Can you work these out from the model? Positions are in its coordinate system, mm. Face numbers are marked on the shaded views. A direction names the side the tool comes from. Give positions to 0.01 mm unless a question says otherwise; leave off trailing zeros. Loops run counter-clockwise (first coordinate to the right, second up) from the corner with the lowest first, then second, coordinate; pieces in that order, holes last. Notation, with made-up numbers: (85, 78.5) - (140, 78.5) arc R26 ccw to (140, 96.5) - close; hole circle Ø9 at (-25, 13). An arc over 180 degrees is marked (long way). Answer as a JSON object with one key per item and string values. Group by question number.
Item 1: Please list where these lines run through material, in increasing order: L1, parallel to Y at x = 9, z = 1.5; L2, parallel to Z at x = -45.5, y = -2.5; L3, parallel to Y at x = 9, z = 12.
Item 2: Suppose I cut it at C-C on x = -45.5. Write out the boundary of the cut face in (y, z), and give its area (3 significant figures).
Item 3: Which directions (+Z, -Z, +X, -X, +Y, -Y) give clear straight access to the entire face, cutting with the end or side of a thin tool? Please do the marked faces 1 and 2.
Item 4: Suppose I cut it at D-D on y = 13. Write out the boundary of the cut face in (x, z), and give its area (3 significant figures).
Item 5: Suppose I cut it at B-B on x = 20.5. Write out the boundary of the cut face in (y, z).
Item 6: Suppose I cut it at A-A on z = 26. Write out the boundary of the cut face in (x, y).
Item 7: Thinking about a two-plate mould opening in Y: for the marked faces 3, 4 and 5, which applies, pulls with the +Y half, pulls with the -Y half, needs draft (parallel to the pull), parting line crosses it, or undercut?
Item 8: Will these pins go through, and if not, where does the flat tip stop? pin 1 (6 mm diameter, centred on x = 16.5, z = 27, fed in from -Y); pin 2 (8 mm diameter, centred on x = -36, z = 26.5, fed in from +Y); pin 3 (1.5 mm diameter, centred on x = -15, y = -35, fed in from +Z).
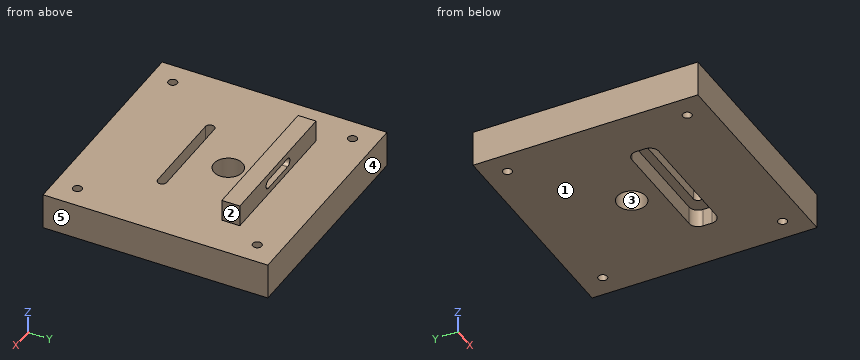
from build123d import *

# Parameters (mm, degrees)
SKETCH1_W           = 125
SKETCH1_H           = 125
BOSS_EXTRUDE1_DEPTH = 20
SKETCH2_R           = 2.5
CUT_EXTRUDE1_DEPTH  = 95.375743383
SKETCH3_R           = 8
CUT_EXTRUDE2_DEPTH  = 95.375743383
SKETCH4_W           = 70
SKETCH4_H           = 15
CUT_EXTRUDE3_DEPTH  = 10
FILLET1_R           = 5
SKETCH6_W           = 80
SKETCH6_H           = 10
BOSS_EXTRUDE2_DEPTH = 12
CUT_EXTRUDE4_DEPTH  = 123.375593875


with BuildPart() as part:
    # Sketch1 → Boss-Extrude1 (new body)
    with BuildSketch(Plane.XY):
        with Locations((4.174852652, 1.227897839)):
            Rectangle(SKETCH1_W, SKETCH1_H)
    extrude(amount=BOSS_EXTRUDE1_DEPTH)

    # Sketch2 → Cut-Extrude1 (cut, through all)
    with BuildSketch(Plane.XY.offset(20)):
        with Locations((-45.825147348, 51.227897839)):
            Circle(SKETCH2_R)
        with Locations((54.174852652, 51.227897839)):
            Circle(SKETCH2_R)
        with Locations((54.174852652, -48.772102161)):
            Circle(SKETCH2_R)
        with Locations((-45.825147348, -48.772102161)):
            Circle(SKETCH2_R)
    extrude(amount=-CUT_EXTRUDE1_DEPTH, mode=Mode.SUBTRACT)

    # Sketch3 → Cut-Extrude2 (cut, through all)
    with BuildSketch(Plane.XY.offset(20)):
        with Locations((4.174852652, 8.627897839)):
            Circle(SKETCH3_R)
        with BuildLine():
            Line((-20.825147348, -12.372102161), (29.174852652, -12.372102161))
            ThreePointArc((29.174852652, -12.372102161), (31.674852652, -14.872102161), (29.174852652, -17.372102161))
            Line((29.174852652, -17.372102161), (-20.825147348, -17.372102161))
            ThreePointArc((-20.825147348, -17.372102161), (-23.325147348, -14.872102161), (-20.825147348, -12.372102161))
        make_face()
    extrude(amount=-CUT_EXTRUDE2_DEPTH, mode=Mode.SUBTRACT)

    # Sketch4 → Cut-Extrude3 (cut)
    with BuildSketch(Plane(origin=(0, 0, 0), x_dir=(-1, 0, 0), z_dir=(0, 0, -1))):
        with Locations((-4.174852652, -14.872102161)):
            Rectangle(SKETCH4_W, SKETCH4_H)
    extrude(amount=-CUT_EXTRUDE3_DEPTH, mode=Mode.SUBTRACT)

    # Fillet1
    fillet1_edges = [part.edges().sort_by_distance(p)[0] for p in [
        (39.174852652, -22.372102161, 5),
        (39.174852652, -7.372102161, 5),
        (-30.825147348, -7.372102161, 5),
        (-30.825147348, -22.372102161, 5),
    ]]
    fillet(fillet1_edges, radius=FILLET1_R)

    # Sketch6 → Boss-Extrude2 (add)
    with BuildSketch(Plane.XY.offset(20)):
        with Locations((4.174852652, 31.227897839)):
            Rectangle(SKETCH6_W, SKETCH6_H)
    extrude(amount=BOSS_EXTRUDE2_DEPTH)

    # Sketch7 → Cut-Extrude4 (cut, through all)
    with BuildSketch(Plane(origin=(0, 36.227897839, 0), x_dir=(1, 0, 0), z_dir=(0, 1, 0))):
        with BuildLine():
            Line((-5.825147348, -28.5), (14.174852652, -28.5))
            ThreePointArc((14.174852652, -28.5), (16.674852652, -26), (14.174852652, -23.5))
            Line((14.174852652, -23.5), (-5.825147348, -23.5))
            ThreePointArc((-5.825147348, -23.5), (-8.325147348, -26), (-5.825147348, -28.5))
        make_face()
    extrude(amount=-CUT_EXTRUDE4_DEPTH, mode=Mode.SUBTRACT)


solid = part.part
Worked out:
{
 "1": {"L1": "y = -61.27 to -22.37, -7.37 to 2.25, 15.01 to 63.73", "L2": "z = 0 to 20", "L3": "y = -61.27 to -17.37, -12.37 to 2.25, 15.01 to 63.73"},
 "2": {"outline": "(-61.27, 0) - (-51.25, 0) - (-51.25, 20) - (-61.27, 20) - close; (-46.29, 0) - (48.75, 0) - (48.75, 20) - (-46.29, 20) - close; (53.71, 0) - (63.73, 0) - (63.73, 20) - (53.71, 20) - close", "area": "2,300 mm2"},
 "3": {"face 1": "-Z, +X, -X, +Y, -Y", "face 2": "+Z, +X, +Y, -Y"},
 "4": {"outline": "(-58.33, 0) - (-2.52, 0) - (-2.52, 20) - (-58.33, 20) - close; (10.87, 0) - (66.67, 0) - (66.67, 20) - (10.87, 20) - close", "area": "2,230 mm2"},
 "5": {"outline": "(-61.27, 0) - (-22.37, 0) - (-22.37, 10) - (-17.37, 10) - (-17.37, 20) - (-61.27, 20) - close; (-12.37, 10) - (-7.37, 10) - (-7.37, 0) - (63.73, 0) - (63.73, 20) - (36.23, 20) - (36.23, 32) - (26.23, 32) - (26.23, 20) - (-12.37, 20) - close"},
 "6": {"outline": "(-35.83, 26.23) - (-8.33, 26.23) - (-8.33, 36.23) - (-35.83, 36.23) - close; (16.67, 26.23) - (44.17, 26.23) - (44.17, 36.23) - (16.67, 36.23) - close"},
 "7": {"face 3": "undercut", "face 4": "pulls with the +Y half", "face 5": "needs draft"},
 "8": {"pin 1": "stops at y = 26.23", "pin 2": "stops at y = 36.23", "pin 3": "stops at z = 20"}
}
